Can you work these out from the model? Positions are in its coordinate system, mm. A direction names the side the tool comes from. Round coordinates to 2 decimals unless told otherwise and drop trailing zeros. Order: outer loops, then holes, each group sorted by start corner. A loop starts at its lowest first (then second) coordinate and runs counter-clockwise, first axis right, second up. Notation, with made-up numbers: (21.25, 14) - (69.25, 14) arc R18 cw to (69.25, 36) - close; hole circle Ø1 at (-7, 47.5). An arc over 180 degrees is marked (long way). Write item = value, one per line.
from build123d import *

# Parameters (mm, degrees)
PAD_DEPTH    = 10
SKETCH001_R  = 2.5
POCKET_DEPTH = 40.001


with BuildPart() as part:
    # Sketch → Pad (new body)
    with BuildSketch(Plane.XY):
        with BuildLine():
            Line((-20, 170), (20, 170))
            Line((20, 170), (20, -30))
            Line((20, -30), (1.5, -30))
            Line((1.5, -9.88686), (1.5, -30))
            ThreePointArc((1.5, -9.88686), (0, 10), (-1.5, -9.88686))
            Line((-1.5, -9.88686), (-1.5, -30))
            Line((-1.5, -30), (-20, -30))
            Line((-20, -30), (-20, 170))
        make_face()
        with BuildLine():
            ThreePointArc((6, 145), (0, 151), (-6, 145))
            Line((-6, 25), (-6, 145))
            ThreePointArc((-6, 25), (0, 19), (6, 25))
            Line((6, 25), (6, 145))
        make_face(mode=Mode.SUBTRACT)
    extrude(amount=PAD_DEPTH)

    # Sketch001 (on Face8 of Pad) → Pocket (cut, through all)
    with BuildSketch(Plane(origin=(-20, 0, 0), x_dir=(0, -1, 0), z_dir=(-1, 0, 0))):
        with Locations((20, 5)):
            Circle(SKETCH001_R)
    extrude(amount=-POCKET_DEPTH, mode=Mode.SUBTRACT)


solid = part.part
(1) If we section it at A-A (z = 5): Write out the boundary of the cut face in (x, y).
Computed:
outline = (-20, -30) - (-1.5, -30) - (-1.5, -22.5) - (-20, -22.5) - close; (-20, -17.5) - (-1.5, -17.5) - (-1.5, -9.89) arc R10 cw (long way) to (1.5, -9.89) - (1.5, -17.5) - (20, -17.5) - (20, 170) - (-20, 170) - close; (1.5, -30) - (20, -30) - (20, -22.5) - (1.5, -22.5) - close; hole (-6, 25) arc R6 ccw to (6, 25) - (6, 145) arc R6 ccw to (-6, 145) - close
(2) Will this pin go through, and if not, where does the flat tip stop? P1, Ø6, axis at y = -20, z = 5, coming from the +X side.
Computed:
P1 = 20
(3) If we section it at D-D (y = -20): Write out the boundary of the cut face in (x, z).
Computed:
outline = (-20, 0) - (-1.5, 0) - (-1.5, 2.5) - (-20, 2.5) - close; (-20, 7.5) - (-1.5, 7.5) - (-1.5, 10) - (-20, 10) - close; (1.5, 0) - (20, 0) - (20, 2.5) - (1.5, 2.5) - close; (1.5, 7.5) - (20, 7.5) - (20, 10) - (1.5, 10) - close
(4) If I drill on line 1 (X direction, y = 32.5, z = 3.25); line 2 (Y direction, x = 0, z = 3); line 3 (Y direction, x = -3, z = 5.5), over which ranges is the centre line in solid material (lowest first)? Write a range as from..to.
Computed:
line_1 = -20..-6, 6..20
line_2 = 10..19, 151..170
line_3 = -30..-22.45, -17.55..-9.54, 9.54..19.8, 150.2..170
(5) If we section it at C-C (x = 4): Write out the boundary of the cut face in (y, z).
Computed:
outline = (-30, 0) - (-9.17, 0) - (-9.17, 10) - (-30, 10) - close; (9.17, 0) - (20.53, 0) - (20.53, 10) - (9.17, 10) - close; (149.47, 0) - (170, 0) - (170, 10) - (149.47, 10) - close; hole circle Ø5 at (-20, 5)
(6) On a 3-axis mill with a long thin cutter (end or side, diameter ignored), from which of +Z, -Z, +X, -X, +Y, -Y can I reach the whole of each face in a straight line? I mean faces 4 (the face through (10.6, -17.5, 5.1)), 5 (the face through (0, 151, 5)), 6 (the face through (1.5, -17.6, 3.8)). Say none if no direction works.
Computed:
face_4 = +X, -X
face_5 = +Z, -Z
face_6 = +Z, -Z, -Y
(7) If we section it at B-B (y = 135): Write out the boundary of the cut face in (x, z).
Computed:
outline = (-20, 0) - (-6, 0) - (-6, 10) - (-20, 10) - close; (6, 0) - (20, 0) - (20, 10) - (6, 10) - close
(8) Thinking about a two-plate mould opening in Y: for faces 1 (the face through (6, 84, 5)), 2 (the face through (-1.5, -17.6, 3.8)), 3 (the face through (-11, -30, 5)), which applies, +Y half, -Y half, draft (parallel to the pull), parting line (faces both ways), or undercut?
Computed:
face_1 = undercut
face_2 = draft
face_3 = -Y half
